Work out the finished part from the listing and answer in its coordinate system (mm). A direction names the side the tool comes from. Round coordinates to 2 decimals unless told otherwise and drop trailing zeros. Write each loop counter-clockwise with the first axis right and the second up, starting at its lowest first coordinate (ties: lowest second). Pieces come first, ordered by that corner, then holes. Notation, with made-up numbers: (-14, 36) - (3, 36) arc R26 ccw to (3, 57) - close; hole circle Ø7 at (6.5, 5.5). An arc over 180 degrees is marked (long way). Write item = value, one per line. Start each with the question number.
from build123d import *

# Parameters (mm, degrees)
F1_DEPTH = 5
F2_DEPTH = 12.7
F3_DEPTH = 2


with BuildPart() as f1:
    # F0 (on Front) → F1 (new body)
    with BuildSketch(Plane.XZ):
        with BuildLine():
            ThreePointArc((39.432288, -47.378316), (40.00265, -47.756794), (40.569589, -48.140379))
            ThreePointArc((40.569589, -48.140379), (13.513407, -32.581288), (-17.696093, -32.282251))
            ThreePointArc((-17.696093, -32.282251), (-33.551282, -38.724603), (-47.021789, -49.280947))
            ThreePointArc((-47.021789, -49.280947), (-46.46503, -48.882729), (-45.904716, -48.489528))
            ThreePointArc((-45.904716, -48.489528), (-3.406376, -34.866086), (39.432288, -47.378316))
        make_face()
        with BuildLine():
            ThreePointArc((-47.932388, 45.724251), (-47.623421, 45.113689), (-47.318573, 44.50106))
            ThreePointArc((-47.318573, 44.50106), (-36.833831, -1.179528), (-47.969069, -46.70592))
            ThreePointArc((-47.969069, -46.70592), (-48.282623, -47.314139), (-48.600267, -47.920232))
            ThreePointArc((-48.600267, -47.920232), (-31.75396, -1.215758), (-47.932388, 45.724251))
        make_face()
        with BuildLine():
            ThreePointArc((-17.705524, 31.319402), (13.504642, 31.692077), (40.590774, 47.201906))
            ThreePointArc((40.590774, 47.201906), (40.026445, 46.814491), (39.458658, 46.43216))
            ThreePointArc((39.458658, 46.43216), (-2.818066, 33.628679), (-45.09479, 46.43216))
            ThreePointArc((-45.09479, 46.43216), (-45.662576, 46.814491), (-46.226906, 47.201906))
            ThreePointArc((-46.226906, 47.201906), (-33.028628, 37.3528), (-17.705524, 31.319402))
        make_face()
        with BuildLine():
            ThreePointArc((41.682442, 44.50106), (41.987289, 45.113689), (42.296256, 45.724251))
            ThreePointArc((42.296256, 45.724251), (25.839489, -0.454927), (42.296256, -46.634105))
            ThreePointArc((42.296256, -46.634105), (41.987289, -46.023543), (41.682442, -45.410914))
            ThreePointArc((41.682442, -45.410914), (31.195115, -0.454927), (41.682442, 44.50106))
        make_face()
        with BuildLine():
            ThreePointArc((-18.227816, 27.025968), (-20.390359, 29.467524), (-17.705524, 31.319402))
            ThreePointArc((-17.705524, 31.319402), (-33.028628, 37.3528), (-46.226906, 47.201906))
            Line((-46.226906, 47.201906), (-47.932388, 45.724251))
            ThreePointArc((-47.932388, 45.724251), (-31.75396, -1.215758), (-48.600267, -47.920232))
            Line((-48.600267, -47.920232), (-47.021789, -49.280947))
            ThreePointArc((-47.021789, -49.280947), (-33.551282, -38.724603), (-17.696093, -32.282251))
            ThreePointArc((-17.696093, -32.282251), (-20.389766, -30.437547), (-18.227816, -27.991167))
            Line((-18.227816, -27.991167), (-18.227816, 27.025968))
        make_face()
        with BuildLine():
            ThreePointArc((42.296256, -46.634105), (25.839489, -0.454927), (42.296256, 45.724251))
            Line((42.296256, 45.724251), (40.590774, 47.201906))
            ThreePointArc((40.590774, 47.201906), (13.504642, 31.692077), (-17.705524, 31.319402))
            ThreePointArc((-17.705524, 31.319402), (-16.512648, 30.547582), (-16.04933, 29.204453))
            Line((-16.04933, 29.204453), (13.037413, 29.204453))
            ThreePointArc((13.037413, 29.204453), (15.215898, 31.382938), (17.394383, 29.204453))
            ThreePointArc((17.394383, 29.204453), (16.75632, 27.664031), (15.215898, 27.025968))
            Line((15.215898, 27.025968), (15.215898, -27.991167))
            ThreePointArc((15.215898, -27.991167), (16.75632, -28.629231), (17.394383, -30.169653))
            ThreePointArc((17.394383, -30.169653), (15.215898, -32.348138), (13.037413, -30.169653))
            Line((13.037413, -30.169653), (-16.04933, -30.169653))
            ThreePointArc((-16.04933, -30.169653), (-16.509656, -31.508953), (-17.696093, -32.282251))
            ThreePointArc((-17.696093, -32.282251), (13.513407, -32.581288), (40.569589, -48.140379))
            Line((40.569589, -48.140379), (42.296256, -46.634105))
        make_face()
    extrude(amount=F1_DEPTH)

    # F0 (on Front) → F2 (join)
    with BuildSketch(Plane.XZ):
        with BuildLine():
            ThreePointArc((-46.226906, 47.201906), (-45.662576, 46.814491), (-45.09479, 46.43216))
            ThreePointArc((-45.09479, 46.43216), (-54.78809, 55.348642), (-47.318573, 44.50106))
            ThreePointArc((-47.318573, 44.50106), (-47.623421, 45.113689), (-47.932388, 45.724251))
            ThreePointArc((-47.932388, 45.724251), (-53.886676, 54.319623), (-46.226906, 47.201906))
        make_face()
        with BuildLine():
            ThreePointArc((40.590774, 47.201906), (48.250545, 54.319623), (42.296256, 45.724251))
            ThreePointArc((42.296256, 45.724251), (41.987289, 45.113689), (41.682442, 44.50106))
            ThreePointArc((41.682442, 44.50106), (49.151959, 55.348642), (39.458658, 46.43216))
            ThreePointArc((39.458658, 46.43216), (40.026445, 46.814491), (40.590774, 47.201906))
        make_face()
        with BuildLine():
            ThreePointArc((41.682442, -45.410914), (41.987289, -46.023543), (42.296256, -46.634105))
            ThreePointArc((42.296256, -46.634105), (48.263981, -55.217796), (40.569589, -48.140379))
            ThreePointArc((40.569589, -48.140379), (40.00265, -47.756794), (39.432288, -47.378316))
            ThreePointArc((39.432288, -47.378316), (49.168873, -56.243758), (41.682442, -45.410914))
        make_face()
        with BuildLine():
            ThreePointArc((-47.969069, -46.70592), (-55.509084, -57.519203), (-45.904716, -48.489528))
            ThreePointArc((-45.904716, -48.489528), (-46.46503, -48.882729), (-47.021789, -49.280947))
            ThreePointArc((-47.021789, -49.280947), (-54.610249, -56.487931), (-48.600267, -47.920232))
            ThreePointArc((-48.600267, -47.920232), (-48.282623, -47.314139), (-47.969069, -46.70592))
        make_face()
    extrude(amount=F2_DEPTH)

    # F0 (on Front) → F3 (join)
    with BuildSketch(Plane.XZ):
        with BuildLine():
            Line((13.037413, 29.204453), (-16.04933, 29.204453))
            ThreePointArc((-16.04933, 29.204453), (-16.687394, 27.664031), (-18.227816, 27.025968))
            Line((-18.227816, 27.025968), (-18.227816, -27.991167))
            ThreePointArc((-18.227816, -27.991167), (-16.687394, -28.629231), (-16.04933, -30.169653))
            Line((-16.04933, -30.169653), (13.037413, -30.169653))
            ThreePointArc((13.037413, -30.169653), (13.675476, -28.629231), (15.215898, -27.991167))
            Line((15.215898, -27.991167), (15.215898, 27.025968))
            ThreePointArc((15.215898, 27.025968), (13.675476, 27.664031), (13.037413, 29.204453))
        make_face()
    extrude(amount=F3_DEPTH)


solid = f1.part
1. For a pull along Z with two mould halves and no side action, classify faces 1 (the face through (-56, -12.7, -55)), 2 (the face through (-55.71, -6.26, -57.34)) as released by +Z, released by -Z, zero draft, split by the parting line, or undercut.
2. Find section A-A on y = -8. Give the vertices of the cut face in (x, z), plus the area to 3 significant figures.
3. Consider line 1 (Z direction, x = -18.5, y = -4.5); line 2 (X direction, y = -1.25, z = 29); line 3 (Z direction, x = -50.5, y = -11). Determine where each line is inside the solid, lowest interval first.
4. Find section C-C on z = -18.5. Give the vertices of the cut face in (x, y).
5. Find section B-B on x = 36.5. Give the vertices of the cut face in (y, z).
6. Which of the six approach directions +Z, -Z, +X, -X, +Y, -Y give full straight-line access (tool end or side, diameter ignored) to faces 3 (the face through (48.423, -6.261, -55.073)), 4 (the face through (-2, -2, 0))?
7. Find section D-D on x = 9.5. Give the vertices of the cut face in (y, z), plus the area to 3 significant figures.
8. Each of these flat-tipped pins is pushed along its axis until it touches: pin 1 (5 mm diameter, centred on x = -6, z = -13.5, fed in from -Y); pin 2 (1.5 mm diameter, centred on x = -8, y = -4, fed in from -Z); pin 3 (1 mm diameter, centred on y = -2, z = -12.5, fed in from -X). Where does it stop, or does it pass through?
Answer key:
q1.face_1 = zero draft
q1.face_2 = undercut
q2.outline = (-48.6, -47.92) arc R101.58 ccw to (-47.97, -46.71) arc R6.63 ccw (long way) to (-45.9, -48.49) arc R76.2 ccw to (-47.02, -49.28) arc R5.26 cw (long way) to start; (-47.93, 45.72) arc R5.26 cw (long way) to (-46.23, 47.2) arc R76.22 ccw to (-45.09, 46.43) arc R6.63 ccw (long way) to (-47.32, 44.5) arc R101.6 ccw to start; (39.43, -47.38) arc R6.63 ccw (long way) to (41.68, -45.41) arc R101.58 ccw to (42.3, -46.63) arc R5.26 cw (long way) to (40.57, -48.14) arc R76.21 ccw to start; (39.46, 46.43) arc R76.21 ccw to (40.59, 47.2) arc R5.26 cw (long way) to (42.3, 45.72) arc R101.58 ccw to (41.68, 44.5) arc R6.63 ccw (long way) to start
q2.area = 190 mm²
q3.line_1 = -36.58 to -32.33, -28.01 to 27.04, 31.37 to 35.26
q3.line_2 = -41.19 to -20.4, -16.06 to 13.05, 17.38 to 35.56
q3.line_3 = -59.1 to -57.72, -47.29 to -45.91, 43.72 to 45.09, 55.6 to 56.97
q4.outline = (-38.45, -5) - (-18.23, -5) - (-18.23, -2) - (15.22, -2) - (15.22, -5) - (32.81, -5) - (32.81, 0) - (-38.45, 0) - close
q5.outline = (-5, -45.55) - (0, -45.55) - (0, -32.86) - (-5, -32.86) - close; (-5, 31.95) - (0, 31.95) - (0, 44.56) - (-5, 44.56) - close
q6.face_3 = +Y, -Y
q6.face_4 = -Y
q7.outline = (-5, -35.8) - (0, -35.8) - (0, 34.63) - (-5, 34.63) - (-5, 29.2) - (-2, 29.2) - (-2, -30.17) - (-5, -30.17) - close
q7.area = 174 mm²
q8.pin_1 = -2
q8.pin_2 = -35.12
q8.pin_3 = -37.61
